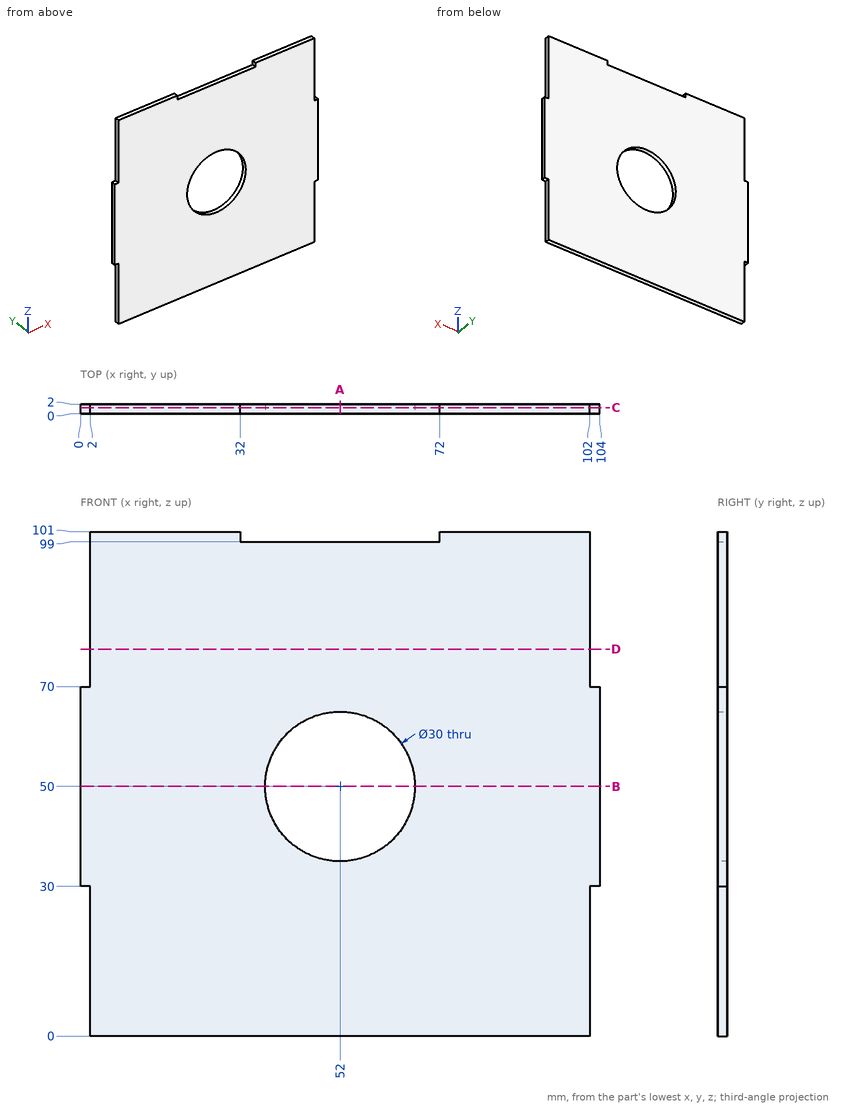
Study the drawing (mm; zero at the part's minimum x, y, z) and answer. Give positions to 0.01 mm unless a question says otherwise; leave off trailing zeros. Order: outer loops, then holes, each group sorted by start corner. A loop starts at its lowest first (then second) coordinate and runs counter-clockwise, first axis right, second up. Notation, with made-up numbers: M 72.25,49 L 104.25,49 A10 cw 104.25,63 Z; hole C -36.75,-34 d11. An arc over 180 degrees is marked long. Put each result on its own line as item: value. Start each with the question number.
Item 1: The part is cut by section C-C, the plane y = 1.25. Determine the outline of the cut face in (x, z).
Item 2: Find the intervals of material crossed by line 1 along X through (y, z) = (0.4, 50); line 2 along Z through (x, y) = (59, 1.7); line 3 along X through (y, z) = (1.4, 72), in increasing order.
Item 3: The part is cut by section D-D, the plane z = 77.5. Determine the outline of the cut face in (x, y).
Item 4: The part is cut by section B-B, the plane z = 50. Determine the outline of the cut face in (x, y), and give its area (3 significant figures).
Item 5: Flat-ended cylindrical pins translate along their axes: P1, Ø1, axis at x = 103.5, y = 1.5, coming from the -Z side; P2, Ø1, axis at y = 1, z = 9.5, coming from the +X side; P3, Ø1, axis at x = 103, y = 1, coming from the +Z side; P4, Ø12, axis at x = 44, z = 48, coming from the -Y side. Find the tip coordinate at first contact, or state that the pin passes through.
Item 6: The part is cut by section A-A, the plane x = 52. Determine the outline of the cut face in (y, z), and give its area (3 significant figures).
Answer key:
1. outline: M 0,30 L 2,30 L 2,0 L 102,0 L 102,30 L 104,30 L 104,70 L 102,70 L 102,101 L 72,101 L 72,99 L 32,99 L 32,101 L 2,101 L 2,70 L 0,70 Z; hole C 52,50 d30
2. line 1: x = 0 to 37, 67 to 104
2. line 2: z = 0 to 36.73, 63.27 to 99
2. line 3: x = 2 to 102
3. outline: M 2,0 L 102,0 L 102,2 L 2,2 Z
4. outline: M 0,0 L 37,0 L 37,2 L 0,2 Z; M 67,0 L 104,0 L 104,2 L 67,2 Z
4. area: 148 mm²
5. P1: stops at z = 30
5. P2: stops at x = 102
5. P3: stops at z = 70
5. P4: passes through
6. outline: M 0,0 L 2,0 L 2,35 L 0,35 Z; M 0,65 L 2,65 L 2,99 L 0,99 Z
6. area: 138 mm²
